Verification items for the finished model (mm, model axes). A direction names the side the tool comes from. Give positions to 0.01 mm unless a question says otherwise; leave off trailing zeros. Write each loop counter-clockwise with the first axis right and the second up, starting at its lowest first coordinate (ties: lowest second). Pieces come first, ordered by that corner, then holes. Notation, with made-up numbers: (27, 60.25) -> (86, 60.25) arc R18 ccw to (86, 84.25) -> close; hole circle Ø9 at (61, 63.5). An arc over 180 degrees is marked (long way). Use one line per item in the form item = value. Start each with the question number.
(1) Scan lines: L1, parallel to Y at x = 54, z = -6.5; L2, parallel to X at y = -5, z = 9; L3, parallel to X at y = -20.5, z = -7.5. Record each from-to range of solid material in increasing order.
(2) Set-up check for faces 4 (the face through (99.149, 1, -1)), 5 (the face through (40, 1, -17.412)), 6 (the face through (62.528, -52.052, -0.485)): record each of +Z, -Z, +X, -X, +Y, -Y from which the full face is reachable in a straight line by a thin tool's end or side.
(3) Section check B-B, the plane x = 79. Record the cut outline in (y, z), plus the area to 3 significant figures.
(4) Section check A-A, the plane z = 14. Record the cut outline in (x, y).
(5) Release check for a two-part mould opening along X. For faces 1 (the face through (41, -50.8, -1)), 2 (the face through (-17.087, -52, -1)), 3 (the face through (24.133, -52.052, 0.381)) record: pulls with the +X half, pulls with the -X half, needs draft (parallel to the pull), parting line crosses it, or undercut.
(6) Section check C-C, the plane x = 0. Record the cut outline in (y, z), plus the area to 3 significant figures.
(7) Depth check by flat-ended pin: pin 1 Ø3.5 at (x, z) = (34.95, 0) entering from -Y; pin 2 Ø3 at (x, y) = (48, -52.5) entering from +Z; pin 3 Ø2 at (x, y) = (13.5, 1.5) entering from -Z; pin 4 Ø10 at (y, z) = (-44.5, -3) entering from -X. Enter the tip coordinate at first touch or a pass-through.
(8) Section check D-D, the plane z = -10. Record the cut outline in (x, y).
from build123d import *

# Parameters (mm, degrees)
F0_R     = 12.7
F1_DEPTH = 50.8
F2_R     = 1.27
F3_DEPTH = 2.54
F4_R     = 1.27
F5_DEPTH = 2.54
F7_DEPTH = 2.54
F8_W     = 116.849138
F8_H     = 33.673273
F8_R     = 1.27
F8_R_2   = 1.267219
F8_R_3   = 1.172691
F9_DEPTH = 2.54


with BuildPart() as f1:
    # F0 (on Front) → F1 (new body)
    with BuildSketch(Plane.XZ):
        Circle(F0_R)
    extrude(amount=F1_DEPTH)

    # F2 (on face) → F3 (join)
    with BuildSketch(Plane.XZ.offset(50.8)):
        Circle(F2_R)
    extrude(amount=F3_DEPTH)

    # F4 (on face) → F5 (join)
    with BuildSketch(Plane(origin=(0, 0, 0), x_dir=(-1, 0, 0), z_dir=(0, 1, 0))):
        Circle(F4_R)
    extrude(amount=F5_DEPTH)

    # F6 (on Front) → F7 (join)
    with BuildSketch(Plane.XZ):
        with BuildLine():
            Line((21.612578, -0.492717), (-17.124444, -0.719515))
            Line((-17.124444, -0.719515), (-17.124444, -17.412249))
            Line((-17.124444, -17.412249), (99.149086, -17.412249))
            Line((99.149086, -17.412249), (99.149086, -0.038756))
            Line((99.149086, -0.038756), (96.968265, -0.051524))
            ThreePointArc((96.968265, -0.051524), (96.968281, -0.055242), (96.968286, -0.05896))
            ThreePointArc((96.968286, -0.05896), (95.702004, -1.328954), (94.428308, -0.066395))
            Line((94.428308, -0.066395), (88.334388, -0.102074))
            ThreePointArc((88.334388, -0.102074), (88.334405, -0.105792), (88.33441, -0.109509))
            ThreePointArc((88.33441, -0.109509), (87.068128, -1.379504), (85.794432, -0.116945))
            Line((85.794432, -0.116945), (76.246966, -0.172843))
            ThreePointArc((76.246966, -0.172843), (76.246982, -0.176561), (76.246987, -0.180279))
            ThreePointArc((76.246987, -0.180279), (74.980705, -1.450273), (73.707009, -0.187714))
            Line((73.707009, -0.187714), (62.143279, -0.255418))
            ThreePointArc((62.143279, -0.255418), (62.143295, -0.259135), (62.143301, -0.262853))
            ThreePointArc((62.143301, -0.262853), (60.877019, -1.532848), (59.603323, -0.270289))
            Line((59.603323, -0.270289), (45.592063, -0.352322))
            ThreePointArc((45.592063, -0.352322), (45.592079, -0.35604), (45.592085, -0.359757))
            ThreePointArc((45.592085, -0.359757), (44.325802, -1.629752), (43.052106, -0.367193))
            Line((43.052106, -0.367193), (35.948796, -0.408781))
            ThreePointArc((35.948796, -0.408781), (35.948813, -0.412499), (35.948818, -0.416217))
            ThreePointArc((35.948818, -0.416217), (34.682536, -1.686211), (33.40884, -0.423652))
            Line((33.40884, -0.423652), (24.152535, -0.477846))
            ThreePointArc((24.152535, -0.477846), (24.152551, -0.481564), (24.152557, -0.485282))
            ThreePointArc((24.152557, -0.485282), (22.886274, -1.755276), (21.612578, -0.492717))
        make_face()
        with BuildLine():
            Line((99.149086, 15.97322), (-17.124444, 15.97322))
            Line((-17.124444, 15.97322), (-17.124444, -0.719515))
            Line((-17.124444, -0.719515), (21.612578, -0.492717))
            ThreePointArc((21.612578, -0.492717), (22.875121, 0.784697), (24.152535, -0.477846))
            Line((24.152535, -0.477846), (33.40884, -0.423652))
            ThreePointArc((33.40884, -0.423652), (34.671383, 0.853761), (35.948796, -0.408781))
            Line((35.948796, -0.408781), (43.052106, -0.367193))
            ThreePointArc((43.052106, -0.367193), (44.314649, 0.910221), (45.592063, -0.352322))
            Line((45.592063, -0.352322), (59.603323, -0.270289))
            ThreePointArc((59.603323, -0.270289), (60.865865, 1.007125), (62.143279, -0.255418))
            Line((62.143279, -0.255418), (73.707009, -0.187714))
            ThreePointArc((73.707009, -0.187714), (74.969552, 1.089699), (76.246966, -0.172843))
            Line((76.246966, -0.172843), (85.794432, -0.116945))
            ThreePointArc((85.794432, -0.116945), (87.056975, 1.160469), (88.334388, -0.102074))
            Line((88.334388, -0.102074), (94.428308, -0.066395))
            ThreePointArc((94.428308, -0.066395), (95.690851, 1.211018), (96.968265, -0.051524))
            Line((96.968265, -0.051524), (99.149086, -0.038756))
            Line((99.149086, -0.038756), (99.149086, 15.97322))
        make_face()
    extrude(amount=-F7_DEPTH)

    # F8 (on face) → F9 (join)
    with BuildSketch(Plane.XZ.offset(50.8)):
        with Locations((41.337759, -0.882761)):
            Rectangle(F8_W, F8_H)
        Circle(F8_R, mode=Mode.SUBTRACT)
        with Locations((22.921631, 0)):
            Circle(F8_R, mode=Mode.SUBTRACT)
        with Locations((34.950949, 0)):
            Circle(F8_R, mode=Mode.SUBTRACT)
        with Locations((44.44854, 0)):
            Circle(F8_R, mode=Mode.SUBTRACT)
        with Locations((61.357126, 0)):
            Circle(F8_R_2, mode=Mode.SUBTRACT)
        with Locations((75.108536, 0)):
            Circle(F8_R_3, mode=Mode.SUBTRACT)
        with Locations((87.163217, 0)):
            Circle(F8_R, mode=Mode.SUBTRACT)
        with Locations((95.73599, 0)):
            Circle(F8_R, mode=Mode.SUBTRACT)
    extrude(amount=F9_DEPTH)


solid = f1.part
Completed:
q1.L1 = -53.34 to -50.8, 0 to 2.54
q1.L2 = -8.96 to 8.96
q1.L3 = -10.25 to 10.25
q2.face_4 = +Z, -Z, +X, +Y
q2.face_5 = -Z, +X, -X, +Y
q2.face_6 = -Y
q3.outline = (-53.34, -17.72) -> (-50.8, -17.72) -> (-50.8, 15.95) -> (-53.34, 15.95) -> close; (0, -17.41) -> (2.54, -17.41) -> (2.54, 15.97) -> (0, 15.97) -> close
q3.area = 170 mm²
q4.outline = (-17.12, 0) -> (99.15, 0) -> (99.15, 2.54) -> (-17.12, 2.54) -> close; (-17.09, -53.34) -> (99.76, -53.34) -> (99.76, -50.8) -> (-17.09, -50.8) -> close
q5.face_1 = needs draft
q5.face_2 = pulls with the -X half
q5.face_3 = undercut
q6.outline = (-53.34, -17.72) -> (-50.8, -17.72) -> (-50.8, -12.7) -> (0, -12.7) -> (0, -17.41) -> (2.54, -17.41) -> (2.54, 15.97) -> (0, 15.97) -> (0, 12.7) -> (-50.8, 12.7) -> (-50.8, 15.95) -> (-53.34, 15.95) -> close
q6.area = 1,460 mm²
q7.pin_1 = -53.34
q7.pin_2 = 15.95
q7.pin_3 = -17.41
q7.pin_4 = -12.7
q8.outline = (-17.12, 0) -> (-7.83, 0) -> (-7.83, -50.8) -> (-17.09, -50.8) -> (-17.09, -53.34) -> (99.76, -53.34) -> (99.76, -50.8) -> (7.83, -50.8) -> (7.83, 0) -> (99.15, 0) -> (99.15, 2.54) -> (-17.12, 2.54) -> close
